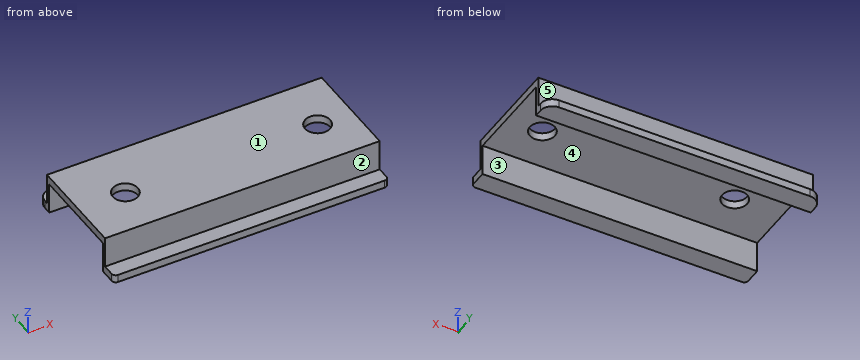
```python
from build123d import *

# Parameters (mm, degrees)
SKETCH_1_W          = 350
SKETCH_1_H          = 170
EXTRUDE_1_DEPTH     = 50
SKETCH_2_W          = 350
SKETCH_2_H          = 20
CUT_EXTRUDE_1_DEPTH = 40
SKETCH_3_W          = 350
SKETCH_3_H          = 120
CUT_EXTRUDE_2_DEPTH = 40
SKETCH_4_R          = 16
CUT_EXTRUDE_3_DEPTH = 227.34896931
FILLET_1_R          = 5
FILLET_2_R          = 5
FILLET_3_R          = 15
FILLET_4_R          = 15


with BuildPart() as part:
    # 草图1 → 凸台-拉伸1 (new body)
    with BuildSketch(Plane.XY):
        with Locations((11.189258312, 33.606138107)):
            Rectangle(SKETCH_1_W, SKETCH_1_H)
    extrude(amount=EXTRUDE_1_DEPTH)

    # 草图2 → 切除-拉伸1 (cut)
    with BuildSketch(Plane.XY.offset(50)):
        with Locations((11.189258312, -41.393861893)):
            Rectangle(SKETCH_2_W, SKETCH_2_H)
        with Locations((11.189258312, 108.606138107)):
            Rectangle(SKETCH_2_W, SKETCH_2_H)
    extrude(amount=-CUT_EXTRUDE_1_DEPTH, mode=Mode.SUBTRACT)

    # 草图3 → 切除-拉伸2 (cut)
    with BuildSketch(Plane(origin=(0, 0, 0), x_dir=(-1, 0, 0), z_dir=(0, 0, -1))):
        with Locations((-11.189258312, 33.606138107)):
            Rectangle(SKETCH_3_W, SKETCH_3_H)
    extrude(amount=-CUT_EXTRUDE_2_DEPTH, mode=Mode.SUBTRACT)

    # 草图4 → 切除-拉伸3 (cut, through all)
    with BuildSketch(Plane.XY.offset(50)):
        with Locations((-103.810741688, 28.606138107)):
            Circle(SKETCH_4_R)
        with Locations((141.189258312, 28.606138107)):
            Circle(SKETCH_4_R)
    extrude(amount=-CUT_EXTRUDE_3_DEPTH, mode=Mode.SUBTRACT)

    # 圆角1
    fillet_1_edges = [part.edges().sort_by_distance(p)[0] for p in [
        (-163.810741688, -51.393861893, 5),
    ]]
    fillet(fillet_1_edges, radius=FILLET_1_R)

    # 圆角2
    fillet_2_edges = [part.edges().sort_by_distance(p)[0] for p in [
        (186.189258312, -51.393861893, 5),
    ]]
    fillet(fillet_2_edges, radius=FILLET_2_R)

    # 圆角3
    fillet_3_edges = [part.edges().sort_by_distance(p)[0] for p in [
        (186.189258312, 118.606138107, 5),
    ]]
    fillet(fillet_3_edges, radius=FILLET_3_R)

    # 圆角4
    fillet_4_edges = [part.edges().sort_by_distance(p)[0] for p in [
        (-163.810741688, 118.606138107, 5),
    ]]
    fillet(fillet_4_edges, radius=FILLET_4_R)


solid = part.part
```
Check sheet for the modelled part. Datum: model origin and axes. Units: mm. Face numbers are marked on the shaded views. A direction names the side the tool comes from. Coordinates: 2 decimals unless noted, no trailing zeros. Write each loop counter-clockwise with the first axis right and the second up, starting at its lowest first coordinate (ties: lowest second). Pieces come first, ordered by that corner, then holes. Notation, with made-up numbers: M 56.5,72.5 L 105.5,72.5 A29 ccw 105.5,110.5 Z; hole C -12.5,51 d11. An arc over 180 degrees is marked long. Write item = value, one per line. Start each with the question number.
1. Thickness scan on probe 1 along Y at (x, z) = (-107.5, 30.5); probe 2 along Y at (x, z) = (2, 7); probe 3 along Z at (x, y) = (-136, 107). Record the ranges inside material, lowest first.
2. Sectioned sample at D-D (x = 58). Record the cut outline in (y, z), then the cut area to 3 significant figures.
3. Tool access check on the marked faces 4 and 5. Record the directions out of +Z, -Z, +X, -X, +Y, -Y that give a thin tool (end or side, any length) a straight path to the whole face; none if there is none.
4. Mould release check, pull along Y, two halves, no side actions. Record for the marked faces 1, 2 and 3: pulls with the +Y half, pulls with the -Y half, needs draft (parallel to the pull), parting line crosses it, or undercut.
5. Go/stop test with flat-tipped pins: pin 1 (8 mm diameter, centred on x = -26.5, z = 27.5, fed in from +Y); pin 2 (1.5 mm diameter, centred on x = 79, z = 39.5, fed in from -Y); pin 3 (10 mm diameter, centred on x = 48, y = 111, fed in from +Z). Record where each tip stops, or that it passes through.
6. Sectioned sample at A-A (z = 6). Record the cut outline in (x, y), then the cut area to 3 significant figures.
7. Sectioned sample at C-C (y = 23.5). Record the cut outline in (x, z).
8. Sectioned sample at B-B (x = -93.5). Record the cut outline in (y, z), then the cut area to 3 significant figures.
The answers:
q1.probe_1 = -31.39 to -26.39, 93.61 to 98.61
q1.probe_2 = -51.39 to -26.39, 93.61 to 118.61
q1.probe_3 = 0 to 10
q2.outline = M -51.39,0 L -26.39,0 L -26.39,40 L 93.61,40 L 93.61,0 L 118.61,0 L 118.61,10 L 98.61,10 L 98.61,50 L -31.39,50 L -31.39,10 L -51.39,10 Z
q2.area = 2,100 mm²
q3.face_4 = -Z, +X, -X
q3.face_5 = +Z, +X, -X, +Y
q4.face_1 = needs draft
q4.face_2 = pulls with the -Y half
q4.face_3 = undercut
q5.pin_1 = 98.61
q5.pin_2 = -31.39
q5.pin_3 = 10
q6.outline = M -163.81,-46.39 A5 ccw -158.81,-51.39 L 181.19,-51.39 A5 ccw 186.19,-46.39 L 186.19,-26.39 L -163.81,-26.39 Z; M -163.81,93.61 L 186.19,93.61 L 186.19,103.61 A15 ccw 171.19,118.61 L -148.81,118.61 A15 ccw -163.81,103.61 Z
q6.area = 17,400 mm²
q7.outline = M -163.81,40 L -118.97,40 L -118.97,50 L -163.81,50 Z; M -88.65,40 L 126.03,40 L 126.03,50 L -88.65,50 Z; M 156.35,40 L 186.19,40 L 186.19,50 L 156.35,50 Z
q8.outline = M -51.39,0 L -26.39,0 L -26.39,40 L 16.37,40 L 16.37,50 L -31.39,50 L -31.39,10 L -51.39,10 Z; M 40.84,40 L 93.61,40 L 93.61,0 L 118.61,0 L 118.61,10 L 98.61,10 L 98.61,50 L 40.84,50 Z
q8.area = 1,860 mm²
